Read the model definition and answer for the solid it produces. Units are mm, in the model's axes. Coordinates: 2 decimals unless noted, no trailing zeros. Write each loop counter-clockwise with the first axis right and the second up, starting at its lowest first coordinate (ties: lowest second). Pieces come first, ordered by that corner, then holes.
(1) The part is cut by section B-B, the plane y = -6. Determine the outline of the cut face in (x, z) (3 decimals), and give its area (3 significant figures).
(2) Given pin 1 (2 mm diameter, centred on x = -67.5, z = 5, fed in from +Y); pin 2 (5 mm diameter, centred on x = -144, z = 7, fed in from -Y); pin 3 (3 mm diameter, centred on x = -131, z = 3.5, fed in from -Y), each flat-ended and moving along its own axis, determine where each tip first touches the part or whether it passes through.
(3) The part is cut by section A-A, the plane z = 8. State how many separate pieces and enclosed holes the cut face has, and give its area (3 significant figures).
(4) Straight lines are drawn through the part: line 1 along X through (y, z) = (55.5, 6) (3 decimals); line 2 along Y through (x, z) = (-20.5, 3.5) (3 decimals); line 3 along X through (y, z) = (-64.5, 7.25). For each, find the intervals that lie inside material, in ascending order.
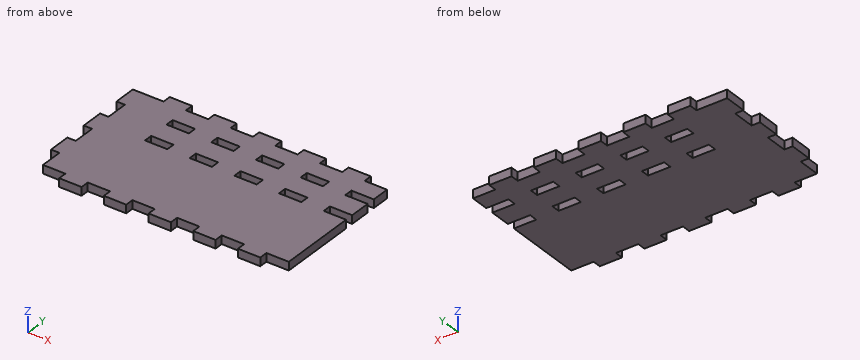
```python
from build123d import *

# Parameters (mm, degrees)
SKETCH1_W               = 279.4
SKETCH1_H               = 152.4
BOSS_EXTRUDE1_DEPTH     = 9.525
SKETCH2_W               = 25.4
SKETCH2_H               = 9.525
BOSS_EXTRUDE2_DEPTH     = 9.525
LPATTERN1_COUNT         = 5
LPATTERN1_PITCH         = 50.8
MIRROR1_COPY_1_SKETCH_W = 25.4
MIRROR1_COPY_1_SKETCH_H = 9.525
MIRROR1_COPY_1_DEPTH    = 9.525
MIRROR1_COPY_2_SKETCH_W = 25.4
MIRROR1_COPY_2_SKETCH_H = 9.525
MIRROR1_COPY_2_DEPTH    = 9.525
MIRROR1_COPY_3_SKETCH_W = 25.4
MIRROR1_COPY_3_SKETCH_H = 9.525
MIRROR1_COPY_3_DEPTH    = 9.525
MIRROR1_COPY_4_SKETCH_W = 25.4
MIRROR1_COPY_4_SKETCH_H = 9.525
MIRROR1_COPY_4_DEPTH    = 9.525
SKETCH3_W               = 9.525
SKETCH3_H               = 25.4
BOSS_EXTRUDE3_DEPTH     = 9.525
LPATTERN2_COUNT         = 3
LPATTERN2_PITCH         = 50.8
SKETCH4_W               = 25.4
SKETCH4_H               = 9.525
CUT_EXTRUDE1_DEPTH      = 10.525
LPATTERN3_COUNT         = 5
LPATTERN3_PITCH         = 50.8
SKETCH5_W               = 25.4
SKETCH5_H               = 9.525
CUT_EXTRUDE2_DEPTH      = 10.525
LPATTERN4_COUNT         = 5
LPATTERN4_PITCH         = 50.8


with BuildPart() as part:
    # Sketch1 → Boss-Extrude1 (new body)
    with BuildSketch(Plane.XY):
        Rectangle(SKETCH1_W, SKETCH1_H)
    extrude(amount=BOSS_EXTRUDE1_DEPTH)

    # Sketch2 → Boss-Extrude2 (add)
    with BuildSketch(Plane.XZ.offset(76.2)):
        with Locations((-101.6, 4.7625)):
            Rectangle(SKETCH2_W, SKETCH2_H)
    boss_extrude2 = extrude(amount=BOSS_EXTRUDE2_DEPTH)

    # LPattern1: Boss-Extrude2 ×5
    with Locations(*[(i * LPATTERN1_PITCH, 0, 0) for i in range(1, LPATTERN1_COUNT)]):
        add(boss_extrude2)

    # Mirror1: Boss-Extrude2 across plane
    add(boss_extrude2.mirror(Plane.ZX))

    # Mirror1 copy 1 sketch → Mirror1 copy 1 (add)
    with BuildSketch(Plane(origin=(50.8, 76.2, 0), x_dir=(1, 0, 0), z_dir=(0, 1, 0))):
        with Locations((-101.6, -4.7625)):
            Rectangle(MIRROR1_COPY_1_SKETCH_W, MIRROR1_COPY_1_SKETCH_H)
    extrude(amount=MIRROR1_COPY_1_DEPTH)

    # Mirror1 copy 2 sketch → Mirror1 copy 2 (add)
    with BuildSketch(Plane(origin=(101.6, 76.2, 0), x_dir=(1, 0, 0), z_dir=(0, 1, 0))):
        with Locations((-101.6, -4.7625)):
            Rectangle(MIRROR1_COPY_2_SKETCH_W, MIRROR1_COPY_2_SKETCH_H)
    extrude(amount=MIRROR1_COPY_2_DEPTH)

    # Mirror1 copy 3 sketch → Mirror1 copy 3 (add)
    with BuildSketch(Plane(origin=(152.4, 76.2, 0), x_dir=(1, 0, 0), z_dir=(0, 1, 0))):
        with Locations((-101.6, -4.7625)):
            Rectangle(MIRROR1_COPY_3_SKETCH_W, MIRROR1_COPY_3_SKETCH_H)
    extrude(amount=MIRROR1_COPY_3_DEPTH)

    # Mirror1 copy 4 sketch → Mirror1 copy 4 (add)
    with BuildSketch(Plane(origin=(203.2, 76.2, 0), x_dir=(1, 0, 0), z_dir=(0, 1, 0))):
        with Locations((-101.6, -4.7625)):
            Rectangle(MIRROR1_COPY_4_SKETCH_W, MIRROR1_COPY_4_SKETCH_H)
    extrude(amount=MIRROR1_COPY_4_DEPTH)

    # Sketch3 → Boss-Extrude3 (add)
    with BuildSketch(Plane.ZY.offset(139.7)):
        with Locations((4.7625, 63.5)):
            Rectangle(SKETCH3_W, SKETCH3_H)
    boss_extrude3 = extrude(amount=BOSS_EXTRUDE3_DEPTH)

    # LPattern2: Boss-Extrude3 ×3
    with Locations(*[(0, -i * LPATTERN2_PITCH, 0) for i in range(1, LPATTERN2_COUNT)]):
        add(boss_extrude3)

    # Sketch4 → Cut-Extrude1 (cut, through all)
    with BuildSketch(Plane(origin=(0, 0, 0), x_dir=(-1, 0, 0), z_dir=(0, 0, -1))):
        with Locations((-127, 17.4625)):
            Rectangle(SKETCH4_W, SKETCH4_H)
    cut_extrude1 = extrude(amount=-CUT_EXTRUDE1_DEPTH, mode=Mode.SUBTRACT)

    # LPattern3: Cut-Extrude1 ×5
    with Locations(*[(-i * LPATTERN3_PITCH, 0, 0) for i in range(1, LPATTERN3_COUNT)]):
        add(cut_extrude1, mode=Mode.SUBTRACT)

    # Sketch5 → Cut-Extrude2 (cut, through all)
    with BuildSketch(Plane.XY.offset(9.525)):
        with Locations((-76.2, 50.905277904)):
            Rectangle(SKETCH5_W, SKETCH5_H)
    cut_extrude2 = extrude(amount=-CUT_EXTRUDE2_DEPTH, mode=Mode.SUBTRACT)

    # LPattern4: Cut-Extrude2 ×5
    with Locations(*[(i * LPATTERN4_PITCH, 0, 0) for i in range(1, LPATTERN4_COUNT)]):
        add(cut_extrude2, mode=Mode.SUBTRACT)


solid = part.part
```
Computed:
1. outline: (-139.7, 0) - (139.7, 0) - (139.7, 9.525) - (-139.7, 9.525) - close
1. area: 2,660 mm2
2. pin 1: stops at y = 76.2
2. pin 2: stops at y = -50.8
2. pin 3: stops at y = -76.2
3. separate pieces: 1
3. enclosed holes: 8
3. area: 43,300 mm2
4. line 1: x = -149.225 to -88.9, -63.5 to -38.1, -12.7 to 12.7, 38.1 to 63.5, 88.9 to 114.3
4. line 2: y = -76.2 to 12.7, 22.225 to 46.143, 55.668 to 76.2
4. line 3: x = -139.7 to 139.7
